Autodesk Inventor part; units mm, degrees
ref_plane "YZ Plane" through (0, 0, 0) normal (1, 0, 0) x (0, 1, 0)
ref_plane "XZ Plane" through (0, 0, 0) normal (0, 1, 0) x (-1, 0, 0)
ref_plane "XY Plane" through (0, 0, 0) normal (0, 0, 1) x (1, 0, 0)
sketch "Sketch1" plane through (0, 0, 0) normal (0, 1, 0) x (-1, 0, 0)
  line L0 (19.05, -215.9) -> (-19.05, -215.9)
  line L1 (-19.05, -215.9) -> (-57.15, -69.85)
  line L2 (19.05, -215.9) -> (57.15, -69.85)
  line L3 (57.15, -69.85) -> (19.05, 0)
  line L4 (19.05, 0) -> (-19.05, 0)
  line L5 (-19.05, 0) -> (-57.15, -69.85)
  line L6 (57.15, -69.85) -> (-57.15, -69.85) construction
  line L7 (-12.7, -50.8) -> (12.7, -50.8) construction
  line L8 (12.7, -50.8) -> (12.7, 0) construction
  line L9 (12.7, 0) -> (-12.7, 0) construction
  line L10 (-12.7, 0) -> (-12.7, -50.8) construction
  point P0 (0, 0)
  point P1 (0, -215.9)
  point P2 (0, -69.85)
  point P3 (0, 0)
  dimension "d0" = 25.4
  dimension "d1" = 50.8
  dimension "d2" = 6.35
  dimension "d3" = 114.3
  dimension "d4" = 215.9
  dimension "d5" = 19.05
  dimension "d6" = 38.1
extrude "Extrusion1" add sketch "Sketch1" along normal mid plane 6.35
fillet "Fillet1" radius 6.604 4 edges at (57.15, 0, -69.85) (19.05, 0, -215.9) (-19.05, 0, -215.9) (-57.15, 0, -69.85)
fillet "Fillet2" [suppressed]
sketch "Sketch2" plane through (0, 3.175, 0) normal (0, 1, 0) x (1, 0, 0)
  arc A0 (20.3379, 210.963) -> (13.9478, 215.9) centre (13.9478, 209.296) ccw construction
  line L0 (20.3379, 210.963) -> (56.4895, 72.3821) construction
  arc A1 (55.8969, 67.5527) -> (56.4895, 72.3821) centre (50.0993, 70.7151) ccw construction
  line L1 (55.8969, 67.5527) -> (19.05, 0) construction
  line L2 (-19.05, 0) -> (-55.8969, 67.5527) construction
  arc A2 (-56.4895, 72.3821) -> (-55.8969, 67.5527) centre (-50.0993, 70.7151) ccw construction
  line L3 (-56.4895, 72.3821) -> (-20.3379, 210.963) construction
  arc A3 (-13.9478, 215.9) -> (-20.3379, 210.963) centre (-13.9478, 209.296) ccw construction
  line L4 (-13.9478, 215.9) -> (13.9478, 215.9) construction
  line L5 (13.9478, 215.9) -> (-13.9478, 215.9) construction
  line L6 (19.05, 0) -> (-19.05, 0)
  point P0 (0, 44.45)
  point P1 (0, 215.9)
  point P2 (0, 215.9)
hole "Hole1" at (0, 3.175, -44.45) direction (0, -1, 0) diameter 31.75 end through all
chamfer "Chamfer1" distance 9.525 distance2 31.75 2 edges at (19.05, 0, 0) (-19.05, 0, 0) measured on face at (6.35, 1.0583, 0)
fillet "Fillet3" radius 6.604 4 edges at (9.525, 0, 0) (34.2536, 0, -27.8732) (-9.525, 0, 0) (-34.2536, 0, -27.8732)
sketch "Sketch3" plane through (0, 3.175, 0) normal (0, 1, 0) x (1, 0, 0)
  circle A0 centre (0, 44.45) radius 15.875 construction
  arc A1 (20.3379, 210.963) -> (13.9478, 215.9) centre (13.9478, 209.296) ccw construction
  line L0 (20.3379, 210.963) -> (56.4895, 72.3821) construction
  arc A2 (55.8969, 67.5527) -> (56.4895, 72.3821) centre (50.0993, 70.7151) ccw construction
  line L1 (55.8969, 67.5527) -> (34.613, 28.5321) construction
  arc A3 (33.7554, 27.3117) -> (34.613, 28.5321) centre (28.8154, 31.6945) ccw construction
  line L2 (33.7554, 27.3117) -> (11.4957, 2.2213) construction
  arc A4 (6.5556, 0) -> (11.4957, 2.2213) centre (6.5556, 6.604) ccw construction
  line L3 (6.5556, 0) -> (-6.5556, 0) construction
  arc A5 (-11.4957, 2.2213) -> (-6.5556, 0) centre (-6.5556, 6.604) ccw construction
  line L4 (-11.4957, 2.2213) -> (-33.7554, 27.3117) construction
  arc A6 (-34.613, 28.5321) -> (-33.7554, 27.3117) centre (-28.8154, 31.6945) ccw construction
  line L5 (-34.613, 28.5321) -> (-55.8969, 67.5527) construction
  arc A7 (-56.4895, 72.3821) -> (-55.8969, 67.5527) centre (-50.0993, 70.7151) ccw construction
  line L6 (-56.4895, 72.3821) -> (-20.3379, 210.963) construction
  arc A8 (-13.9478, 215.9) -> (-20.3379, 210.963) centre (-13.9478, 209.296) ccw construction
  line L7 (-13.9478, 215.9) -> (13.9478, 215.9) construction
  point P0 (0, 0)
  point P1 (0, 12.7)
  dimension "d24" = 31.75
hole "Hole2" at (0, 3.175, -12.7) direction (0, -1, 0) diameter 5.1054 end through all
equation "\"d23\" = d9"
properties part number "CL4-003" material "Aluminum 6061"
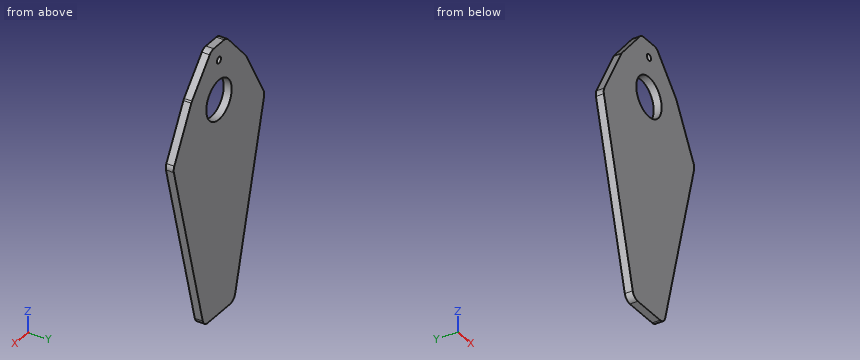
Can you work these out from the model? Positions are in its coordinate system, mm. Coordinates: 2 decimals unless noted, no trailing zeros. Write each loop counter-clockwise with the first axis right and the second up, starting at its lowest first coordinate (ties: lowest second). Pieces come first, ordered by that corner, then holes.
Q1. Imagine slicing it at D-D, the plane x = -48.5. List the corners of the cut face in (y, z) for me (3 decimals).
Results found:
outline: (-3.175, -103.008) - (3.175, -103.008) - (3.175, -53.992) - (-3.175, -53.992) - close
Q2. For P1, Ø1.5, axis at y = 0, z = -170.5, coming from the -X side; P2, Ø2, axis at x = 33, y = -1, coming from the +Z side, each with a flat end and sliding along its axis, tell me the tip position at first contact or that it passes through.
Results found:
P1: stops at x = -31.09
P2: stops at z = -25.33
Q3. Imagine slicing it at C-C, the plane z = -12.7. List the corners of the cut face in (x, y) for me (3 decimals).
Results found:
outline: (-20.792, -3.175) - (-2.553, -3.175) - (-2.553, 3.175) - (-20.792, 3.175) - close; (2.553, -3.175) - (20.792, -3.175) - (20.792, 3.175) - (2.553, 3.175) - close
Q4. Imagine slicing it at A-A, the plane y = -1.75. List the corners of the cut face in (x, z) for me (3 decimals), plus the area to 3 significant figures.
Results found:
outline: (-56.489, -72.382) - (-20.338, -210.963) arc R6.604 ccw to (-13.948, -215.9) - (13.948, -215.9) arc R6.604 ccw to (20.338, -210.963) - (56.489, -72.382) arc R6.604 ccw to (55.897, -67.553) - (34.613, -28.532) arc R6.604 ccw to (33.755, -27.312) - (11.496, -2.221) arc R6.604 ccw to (6.556, 0) - (-6.556, 0) arc R6.604 ccw to (-11.496, -2.221) - (-33.755, -27.312) arc R6.604 ccw to (-34.613, -28.532) - (-55.897, -67.553) arc R6.604 ccw to start; hole circle Ø31.75 at (0, -44.45); hole circle Ø5.105 at (0, -12.7)
area: 15,400 mm2
Q5. Please list where these lines run through material, in increasing order: L1, parallel to Z at x = 0, y = 3 (3 decimals); L2, parallel to Z at x = 12, y = -1; L3, parallel to X at y = 0, z = -44.45 (3 decimals).
Results found:
L1: z = -215.9 to -60.325, -28.575 to -15.253, -10.147 to 0
L2: z = -215.9 to -54.84, -34.06 to -2.79
L3: x = -43.295 to -15.875, 15.875 to 43.295
Q6. Imagine slicing it at B-B, the plane x = 0. List the corners of the cut face in (y, z) for me (3 decimals).
Results found:
outline: (-3.175, -215.9) - (3.175, -215.9) - (3.175, -60.325) - (-3.175, -60.325) - close; (-3.175, -28.575) - (3.175, -28.575) - (3.175, -15.253) - (-3.175, -15.253) - close; (-3.175, -10.147) - (3.175, -10.147) - (3.175, 0) - (-3.175, 0) - close
